Source: CAD feature listing. Evaluate the final solid. Frame: model axes, mm. Face numbers are marked on the shaded views. A direction names the side the tool comes from. Give positions to 0.01 mm unless a question says otherwise; leave off trailing zeros. Order: outer loops, then holes, each group sorted by start corner. A loop starts at its lowest first (then second) coordinate and runs counter-clockwise, first axis right, second up. Notation, with made-up numbers: (-2.75, -6) - (19.25, -6) arc R19 cw to (19.25, 3) - close; hole circle Ø2 at (30.5, -31). An arc over 180 degrees is marked (long way). Use CSV: the item, a comma, the result in double quotes.
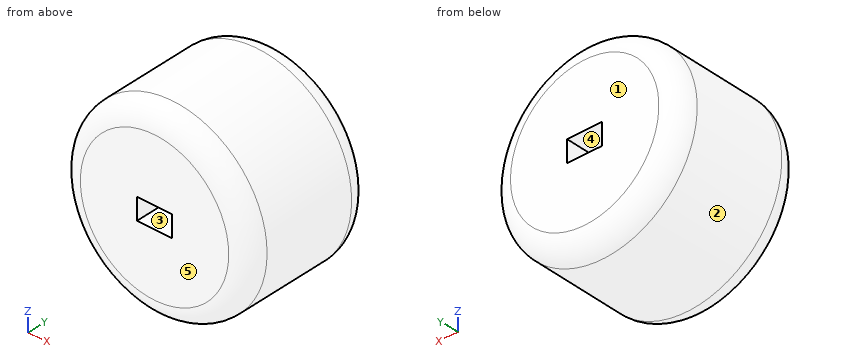
```python
from build123d import *

# Parameters (mm, degrees)
SKETCH2_R           = 14
BOSS_EXTRUDE1_DEPTH = 20
FILLET1_R           = 3
SKETCH3_W           = 5.2
SKETCH3_H           = 3.2
CUT_EXTRUDE1_DEPTH  = 21


with BuildPart() as part:
    # Sketch2 → Boss-Extrude1 (new body)
    with BuildSketch(Plane(origin=(0, 0, 0), x_dir=(1, 0, 0), z_dir=(0, 1, 0))):
        Circle(SKETCH2_R)
    extrude(amount=BOSS_EXTRUDE1_DEPTH)

    # Fillet1
    fillet1_edges = [part.edges().sort_by_distance(p)[0] for p in [
        (-14, 0, 0),
        (-14, 20, 0),
    ]]
    fillet(fillet1_edges, radius=FILLET1_R)

    # Sketch3 → Cut-Extrude1 (cut, through all)
    with BuildSketch(Plane.XZ):
        Rectangle(SKETCH3_W, SKETCH3_H)
    extrude(amount=-CUT_EXTRUDE1_DEPTH, mode=Mode.SUBTRACT)


solid = part.part
```
Item 1: Mould query, pull axis X, two halves, no side actions, for the marked faces 1, 2 and 3. Classes: released by +X, released by -X, zero draft, split by the parting line, or undercut.
Filled in:
face 1,"zero draft"
face 2,"split by the parting line"
face 3,"undercut"
Item 2: Section B-B on z = 0. Return the cut outline in (x, y).
Filled in:
outline,"(-14, 3) arc R3 ccw to (-11, 0) - (-2.6, 0) - (-2.6, 20) - (-11, 20) arc R3 ccw to (-14, 17) - close; (2.6, 0) - (11, 0) arc R3 ccw to (14, 3) - (14, 17) arc R3 ccw to (11, 20) - (2.6, 20) - close"
Item 3: Set-up query: the marked faces 4 and 5. Return all of +Z, -Z, +X, -X, +Y, -Y with unobstructed straight access to the full face (end or side cutting, diameter ignored); none if empty.
Filled in:
face 4,"+Y, -Y"
face 5,"+Z, -Z, +X, -X, -Y"
Item 4: Material intervals for line 1 (Z direction, x = 0, y = 7); line 2 (Y direction, x = -8.75, z = -7); line 3 (X direction, y = 9.75, z = 0.75), sorted ascending. Write a range as from..to.
Filled in:
line 1,"z = -14..-1.6, 1.6..14"
line 2,"y = 0.01..19.99"
line 3,"x = -13.98..-2.6, 2.6..13.98"
Item 5: Section D-D on y = 18.25. Return the cut outline in (x, z), then the cut area to 3 significant figures.
Filled in:
outline,"circle Ø27.45 at (0, 0); hole (-2.6, -1.6) - (2.6, -1.6) - (2.6, 1.6) - (-2.6, 1.6) - close"
area,"575 mm2"
Item 6: Section A-A on x = 0. Return the cut outline in (y, z), then the cut area to 3 significant figures.
Filled in:
outline,"(0, -11) arc R3 ccw to (3, -14) - (17, -14) arc R3 ccw to (20, -11) - (20, -1.6) - (0, -1.6) - close; (0, 1.6) - (20, 1.6) - (20, 11) arc R3 ccw to (17, 14) - (3, 14) arc R3 ccw to (0, 11) - close"
area,"488 mm2"
Item 7: First-contact query: pin 1 (1.5 mm diameter, centred on x = -11, y = 16, fed in from -Z); pin 2 (4 mm diameter, centred on y = 2.5, z = -7.5, fed in from +X); pin 3 (1 mm diameter, centred on y = 13, z = 4, fed in from +X). Flat tips, straight axial feed; report the tip coordinate or a pass-through.
Filled in:
pin 1,"stops at z = -9.54"
pin 2,"stops at x = 12.86"
pin 3,"stops at x = 13.56"
Item 8: Section C-C on y = 12.5. Return the cut outline in (x, z), then the cut area to 3 significant figures.
Filled in:
outline,"circle Ø28 at (0, 0); hole (-2.6, -1.6) - (2.6, -1.6) - (2.6, 1.6) - (-2.6, 1.6) - close"
area,"599 mm2"
